Read the model definition and answer for the solid it produces. Units are mm, in the model's axes. A direction names the side the tool comes from. Coordinates: 2 decimals unless noted, no trailing zeros. Write each loop counter-clockwise with the first axis right and the second up, starting at its lowest first coordinate (ties: lowest second). Pieces come first, ordered by that corner, then holes. Notation, with made-up numbers: (14, -9.75) -> (49, -9.75) arc R9 ccw to (49, 1.25) -> close; hole circle Ø2 at (-9, 17.25). An arc over 180 degrees is marked (long way). Use CSV: the item, a comma, the result in double quotes. Start each with the question number.
from build123d import *

# Parameters (mm, degrees)
BOSS_EXTRUDE1_DEPTH = 10
FILLET1_R           = 5
FILLET2_R           = 5


with BuildPart() as part:
    # Sketch1 → Boss-Extrude1 (new body)
    with BuildSketch(Plane.XY):
        Polygon((0, 0), (15, 0), (15, 10), (30, 50), (45, 10), (45, 0), (60, 0), (60, 5), (50, 5), (50, 10), (30, 63.333333333), (10, 10), (10, 5), (0, 5), align=None)
    extrude(amount=BOSS_EXTRUDE1_DEPTH)

    # Fillet1
    fillet1_edges = [part.edges().sort_by_distance(p)[0] for p in [
        (30, 50, 5),
    ]]
    fillet(fillet1_edges, radius=FILLET1_R)

    # Fillet2
    fillet2_edges = [part.edges().sort_by_distance(p)[0] for p in [
        (30, 63.333333333, 5),
    ]]
    fillet(fillet2_edges, radius=FILLET2_R)


solid = part.part
1) Each of these flat-tipped pins is pushed along its axis until it touches: pin 1 (1.5 mm diameter, centred on y = 21, z = 2, fed in from -X); pin 2 (2.5 mm diameter, centred on y = 7.5, z = 5.5, fed in from -X); pin 3 (4 mm diameter, centred on y = 8.5, z = 4, fed in from +X); pin 4 (1 mm diameter, centred on x = 18, y = 15.5, fed in from +Z). Where does it stop, or does it pass through?
2) The mould has two halves that part along X. Classify faces 6 (the face through (20.1, 23.6, 4.9)), 7 (the face through (52, 0, 5)), 8 (the face through (42.448, 30.139, 4.93)): pulls with the +X half, pulls with the -X half, needs draft (parallel to the pull), parting line crosses it, or undercut.
3) Which of the six approach directions +Z, -Z, +X, -X, +Y, -Y give full straight-line access (tool end or side, diameter ignored) to faces 1 (the face through (55, 5, 5)), 2 (the face through (39.77, 23.95, 4.93)), 3 (the face through (10, 8, 5)), 4 (the face through (29.915, 54.093, 5.07)), 5 (the face through (7, 0, 5))?
4) Find the intervals of material crossed by line 1 along X through (y, z) = (5.5, 8.25); line 2 along X through (y, z) = (18, 3.5); line 3 along Y through (x, z) = (6, 3.75), in increasing order.
5) Section B-B, the plane z = 9 is taken. Give the vertices of the cut face in (x, y), plus the area to 3 significant figures.
6) Section A-A, the plane y = 24.5 is taken. Give the vertices of the cut face in (x, z).
7) Section D-D, the plane y = 39 is taken. Give the vertices of the cut face in (x, z) (3 decimals).
8) Section C-C, the plane y = 48 is taken. Give the vertices of the cut face in (x, z), plus the area to 3 significant figures.
The answers:
1,pin 1,"stops at x = 13.84"
1,pin 2,"stops at x = 10"
1,pin 3,"stops at x = 50"
1,pin 4,"passes through"
2,face 6,"undercut"
2,face 7,"needs draft"
2,face 8,"pulls with the +X half"
3,face 1,"+Z, -Z, +X, +Y"
3,face 2,"+Z, -Z, -Y"
3,face 3,"+Z, -Z, -X, +Y"
3,face 4,"+Z, -Z, +Y"
3,face 5,"+Z, -Z, +X, -X, -Y"
4,line 1,"x = 10 to 15, 45 to 50"
4,line 2,"x = 13 to 18, 42 to 47"
4,line 3,"y = 0 to 5"
5,outline,"(0, 0) -> (15, 0) -> (15, 10) -> (25.32, 37.52) arc R5 cw to (34.68, 37.52) -> (45, 10) -> (45, 0) -> (60, 0) -> (60, 5) -> (50, 5) -> (50, 10) -> (34.68, 50.85) arc R5 ccw to (25.32, 50.85) -> (10, 10) -> (10, 5) -> (0, 5) -> close"
5,area,"667 mm^2"
6,outline,"(15.44, 0) -> (20.44, 0) -> (20.44, 10) -> (15.44, 10) -> close; (39.56, 0) -> (44.56, 0) -> (44.56, 10) -> (39.56, 10) -> close"
7,outline,"(20.875, 0) -> (26.192, 0) -> (26.192, 10) -> (20.875, 10) -> close; (33.808, 0) -> (39.125, 0) -> (39.125, 10) -> (33.808, 10) -> close"
8,outline,"(24.25, 0) -> (35.75, 0) -> (35.75, 10) -> (24.25, 10) -> close"
8,area,"115 mm^2"
